Geometry: final body of the model. Coordinates: model frame, mm. Give positions to 0.01 mm unless a question says otherwise; leave off trailing zeros. Order: outer loops, then holes, each group sorted by start corner. A loop starts at its lowest first (then second) coordinate and runs counter-clockwise, first axis right, second up. Notation, with made-up numbers: (87.5, 76.5) -> (111.5, 76.5) arc R13 cw to (111.5, 84.5) -> close; hole circle Ø7 at (43.5, -7). An arc over 180 degrees is marked (long way). Write item = value, one per line.
```python
from build123d import *

# Parameters (mm, degrees)
SKETCH2_W                                   = 95
SKETCH2_H                                   = 95
EXTRUDE_H_JD_DEPTH                          = 1100
SKETCH10_W                                  = 10
SKETCH10_H                                  = 95
CUT_SLITS_F_R_STOLPFOT_DEPTH                = 200
CUT_SKRUVH_L_F_R_STOLPFOT_REACH             = 49.5
SKETCH8_R                                   = 6
CUT_SKRUVH_L_F_R_STOLPFOT_DIRECTION_2_REACH = 49.5


with BuildPart() as part:
    # Sketch2 → Extrude h_jd (new body)
    with BuildSketch(Plane(origin=(0, 0, 0), x_dir=(1, 0, 0), z_dir=(0, 1, 0))):
        Rectangle(SKETCH2_W, SKETCH2_H)
    extrude(amount=EXTRUDE_H_JD_DEPTH)

    # Sketch10 → Cut-slits f_r stolpfot (cut)
    with BuildSketch(Plane(origin=(0, 0, 0), x_dir=(-1, 0, 0), z_dir=(0, -1, 0))):
        Rectangle(SKETCH10_W, SKETCH10_H)
    extrude(amount=-CUT_SLITS_F_R_STOLPFOT_DEPTH, mode=Mode.SUBTRACT)

    # Sketch8 → Cut-skruvh_l f_r stolpfot (cut, up to next)
    with BuildSketch(Plane(origin=(0, -97.5, 0), x_dir=(0, 1, 0), z_dir=(-1, 0, 0)), mode=Mode.PRIVATE) as cut_skruvh_l_f_r_stolpfot_sk1:
        with Locations(Location((275, 0, 0), (0, 0, 270))):  # turned: the seam where the file's is
            Circle(SKETCH8_R)
    cut_skruvh_l_f_r_stolpfot_tool1 = extrude(cut_skruvh_l_f_r_stolpfot_sk1.sketch, amount=CUT_SKRUVH_L_F_R_STOLPFOT_REACH, mode=Mode.PRIVATE) & part.part
    add(cut_skruvh_l_f_r_stolpfot_tool1.solids().sort_by_distance((0, 177.5, 0))[0], mode=Mode.SUBTRACT)
    # Sketch8 → Cut-skruvh_l f_r stolpfot (cut, up to next)
    with BuildSketch(Plane(origin=(0, -97.5, 0), x_dir=(0, 1, 0), z_dir=(-1, 0, 0)), mode=Mode.PRIVATE) as cut_skruvh_l_f_r_stolpfot_sk2:
        with Locations(Location((140, 0, 0), (0, 0, 270))):  # turned: the seam where the file's is
            Circle(SKETCH8_R)
    cut_skruvh_l_f_r_stolpfot_tool2 = extrude(cut_skruvh_l_f_r_stolpfot_sk2.sketch, amount=CUT_SKRUVH_L_F_R_STOLPFOT_REACH, mode=Mode.PRIVATE) & part.part
    add(cut_skruvh_l_f_r_stolpfot_tool2.solids().sort_by_distance((0, 42.5, 0))[0], mode=Mode.SUBTRACT)

    # Sketch8 → Cut-skruvh_l f_r stolpfot direction 2 (cut, up to next)
    with BuildSketch(Plane(origin=(0, -97.5, 0), x_dir=(0, 1, 0), z_dir=(-1, 0, 0)), mode=Mode.PRIVATE) as cut_skruvh_l_f_r_stolpfot_direction_2_sk1:
        with Locations(Location((275, 0, 0), (0, 0, 270))):  # turned: the seam where the file's is
            Circle(SKETCH8_R)
    cut_skruvh_l_f_r_stolpfot_direction_2_tool1 = extrude(cut_skruvh_l_f_r_stolpfot_direction_2_sk1.sketch, amount=-CUT_SKRUVH_L_F_R_STOLPFOT_DIRECTION_2_REACH, mode=Mode.PRIVATE) & part.part
    add(cut_skruvh_l_f_r_stolpfot_direction_2_tool1.solids().sort_by_distance((0, 177.5, 0))[0], mode=Mode.SUBTRACT)
    # Sketch8 → Cut-skruvh_l f_r stolpfot direction 2 (cut, up to next)
    with BuildSketch(Plane(origin=(0, -97.5, 0), x_dir=(0, 1, 0), z_dir=(-1, 0, 0)), mode=Mode.PRIVATE) as cut_skruvh_l_f_r_stolpfot_direction_2_sk2:
        with Locations(Location((140, 0, 0), (0, 0, 270))):  # turned: the seam where the file's is
            Circle(SKETCH8_R)
    cut_skruvh_l_f_r_stolpfot_direction_2_tool2 = extrude(cut_skruvh_l_f_r_stolpfot_direction_2_sk2.sketch, amount=-CUT_SKRUVH_L_F_R_STOLPFOT_DIRECTION_2_REACH, mode=Mode.PRIVATE) & part.part
    add(cut_skruvh_l_f_r_stolpfot_direction_2_tool2.solids().sort_by_distance((0, 42.5, 0))[0], mode=Mode.SUBTRACT)


solid = part.part
```
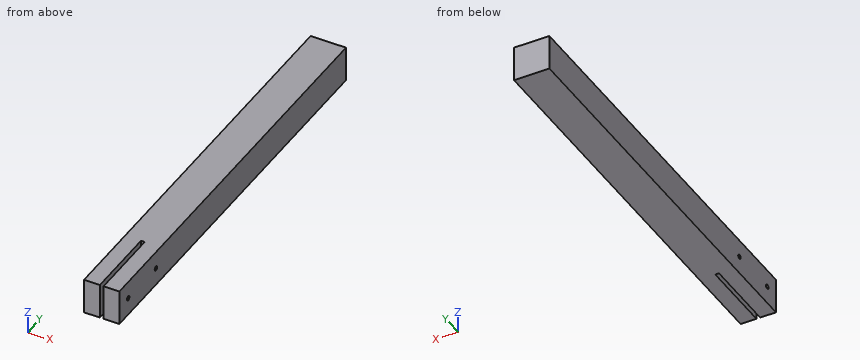
1) Section query A-A (y = 83). Output: boundary loops of the cut face in (x, z), plus the area to 4 significant figures.
Check sheet entries:
outline = (-47.5, -47.5) -> (-5, -47.5) -> (-5, 47.5) -> (-47.5, 47.5) -> close; (5, -47.5) -> (47.5, -47.5) -> (47.5, 47.5) -> (5, 47.5) -> close
area = 8,075 mm²
2) Section query B-B (z = 22). Output: boundary loops of the cut face in (x, y), plus the area to 4 significant figures.
Check sheet entries:
outline = (-47.5, 0) -> (-5, 0) -> (-5, 200) -> (5, 200) -> (5, 0) -> (47.5, 0) -> (47.5, 1100) -> (-47.5, 1100) -> close
area = 102,500 mm²
3) Line query: line 1 (Y direction, x = 32, z = 0); line 2 (Y direction, x = -42.5, z = -1); line 3 (Z direction, x = -32, y = 177.5). Output: solid intervals per line, ascending. Write a range as from..to.
Check sheet entries:
line_1 = 0..36.5, 48.5..171.5, 183.5..1100
line_2 = 0..36.58, 48.42..171.58, 183.42..1100
line_3 = -47.5..-6, 6..47.5
